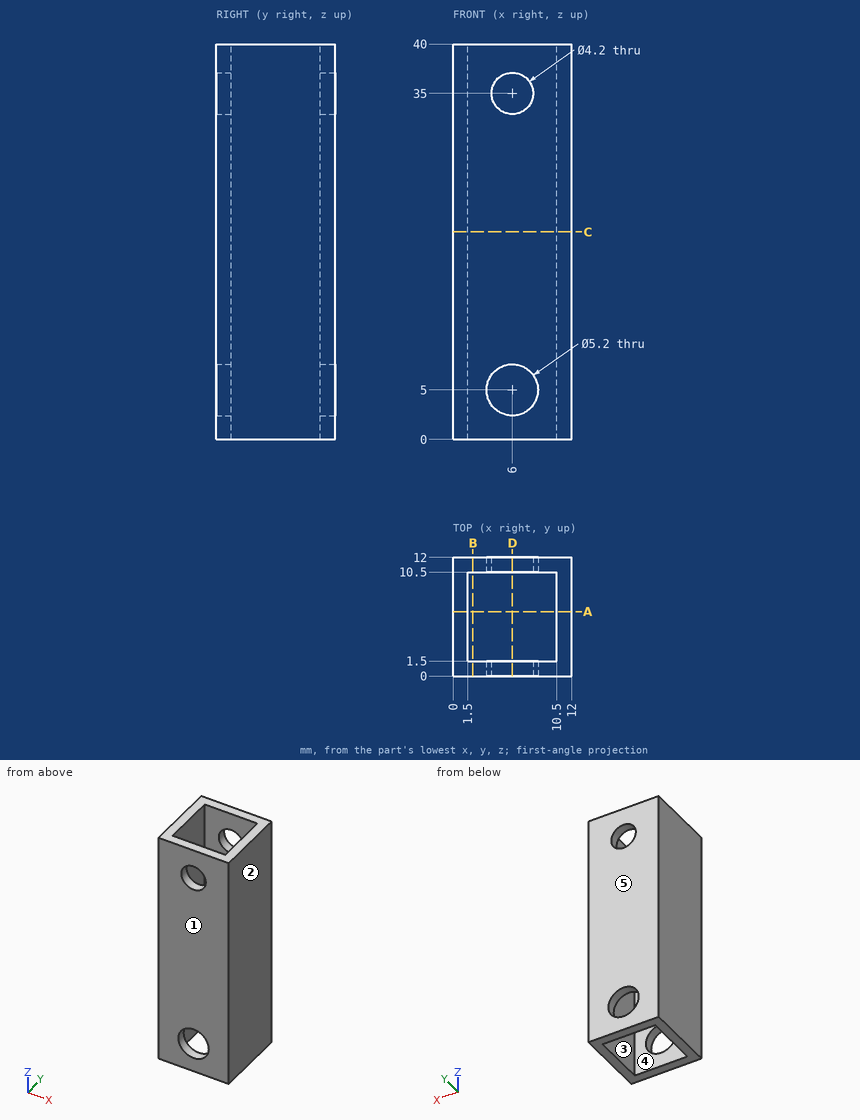
The figure shows three views and two pictorial views of one solid part (mm, origin at its lowest corner). Answer the questions. A direction names the side the tool comes from. Round coordinates to 2 decimals unless told otherwise and drop trailing zeros. Loops run counter-clockwise (first coordinate to the right, second up) from the corner with the lowest first, then second, coordinate; pieces in that order, holes last. Notation, with made-up numbers: M -16,-18 L 34,-18 A22 ccw 34,9 Z; hole C -15,-6 d4. An arc over 180 degrees is marked long. Write each question's results on one line, items separated by ' | '. Start each with the question number.
1) Determine the mould class of the marked faces 1, 2 and 3 for opening direction Y: pulls with the +Y half, pulls with the -Y half, needs draft (parallel to the pull), parting line crosses it, or undercut.
2) Find section C-C on z = 21. Write down the section's boundary in (x, y), plus the area to 3 significant figures.
3) Which of the six approach directions +Z, -Z, +X, -X, +Y, -Y give full straight-line access (tool end or side, diameter ignored) to the marked faces 4 and 5?
4) Straight lines are drawn through the part: probe 1 along Z at (x, y) = (6, 1.2); probe 2 along Y at (x, z) = (9.5, 34). For each, find the intervals that lie inside material, in ascending order.
5) Find section A-A on y = 6.5. Write down the section's boundary in (x, z), plus the area to 3 significant figures.
6) This flat-tipped pin is pushed along its axis until it touches: pin 1 (4 mm diameter, centred on x = 6, z = 35, fed in from -Y). Where does it stop, or does it pass through?
7) Find section D-D on x = 6. Write down the section's boundary in (y, z), plus the area to 3 significant figures.
Final values:
1) face 1: pulls with the -Y half | face 2: needs draft | face 3: undercut
2) outline: M 0,0 L 12,0 L 12,12 L 0,12 Z; hole M 1.5,1.5 L 10.5,1.5 L 10.5,10.5 L 1.5,10.5 Z | area: 63.0 mm²
3) face 4: +Z, -Z | face 5: +Z, -Z, +X, -X, +Y
4) probe 1: 0 to 2.4, 7.6 to 32.9, 37.1 to 40 | probe 2: 0 to 1.5, 10.5 to 12
5) outline: M 0,0 L 1.5,0 L 1.5,40 L 0,40 Z; M 10.5,0 L 12,0 L 12,40 L 10.5,40 Z | area: 120 mm²
6) pin 1: through
7) outline: M 0,0 L 1.5,0 L 1.5,2.4 L 0,2.4 Z; M 0,7.6 L 1.5,7.6 L 1.5,32.9 L 0,32.9 Z; M 0,37.1 L 1.5,37.1 L 1.5,40 L 0,40 Z; M 10.5,0 L 12,0 L 12,2.4 L 10.5,2.4 Z; M 10.5,7.6 L 12,7.6 L 12,32.9 L 10.5,32.9 Z; M 10.5,37.1 L 12,37.1 L 12,40 L 10.5,40 Z | area: 91.8 mm²
